Can you work these out from the model? Positions are in its coordinate system, mm. A direction names the side the tool comes from. Give positions to 0.01 mm unless a question says otherwise; leave off trailing zeros. Write each loop counter-clockwise with the first axis right and the second up, starting at its lowest first coordinate (ties: lowest second). Pieces come first, ordered by that corner, then holes.
1. Thinking about a two-plate mould opening in Z: for faces 3 (the cylindrical face through (-10.74, 1.48, -2.38)), 4 (the flat face through (3, 0, 0)), 5 (the cylindrical face through (-2.44, 6.59, -0.54)), which applies, pulls with the +Z half, pulls with the -Z half, needs draft (parallel to the pull), parting line crosses it, or undercut?
2. If I drill on probe 1 along X at (y, z) = (0.8, 0); probe 2 along Y at (x, z) = (-4, -3.5); probe 3 along X at (y, z) = (11, -1.5), over which ranges is the centre line in solid material (lowest first)?
3. On a 3-axis mill with a long thin cutter (end or side, diameter ignored), from which of +Z, -Z, +X, -X, +Y, -Y can I reach the whole of each face in a straight line? I mean faces 1 (the cylindrical face through (-4.88, 7.93, -1.08)), 2 (the flat face through (-2, 13, 2)). Say none if no direction works.
4. I'm going to push a flat-ended pin straight in: pin 1 (1 mm diameter, centred on y = 1.5, z = -5.5, fed in from -X). Where does the tip first touch, or does it pass through?
5. Suppose I cut it at D-D (y = 1). Please give me the cut outline in (x, z).
6. Suppose I cut it at A-A (z = 0). Please give me the cut outline in (x, y), and give its area (3 significant figures).
7. Suppose I cut it at C-C (z = -8). Please give me the cut outline in (x, y).
8. Suppose I cut it at B-B (x = -8). Please give me the cut outline in (y, z).
```python
from build123d import *

# Parameters (mm, degrees)
SKETCH_1_R          = 11
EXTRUDE_1_DEPTH     = 3
SKETCH_2_R          = 5
EXTRUDE_2_DEPTH     = 10
SKETCH_3_R          = 2.5
CUT_EXTRUDE_1_DEPTH = 13
SKETCH_4_R          = 1.5
CUT_EXTRUDE_2_DEPTH = 3


with BuildPart() as part:
    # 草图1 → 凸台-拉伸1 (new body)
    with BuildSketch(Plane(origin=(0, 0, 0), x_dir=(1, 0, 0), z_dir=(0, 1, 0))):
        with Locations(Location((0, 0, 0), (0, 0, 270))):
            Circle(SKETCH_1_R)
    extrude(amount=EXTRUDE_1_DEPTH)

    # 草图2 → 凸台-拉伸2 (add)
    with BuildSketch(Plane(origin=(0, 3, 0), x_dir=(1, 0, 0), z_dir=(0, 1, 0))):
        with Locations(Location((0, 0, 0), (0, 0, 270))):
            Circle(SKETCH_2_R)
    extrude(amount=EXTRUDE_2_DEPTH)

    # 草图3 → 切除-拉伸1 (cut)
    with BuildSketch(Plane(origin=(0, 13, 0), x_dir=(1, 0, 0), z_dir=(0, 1, 0))):
        with Locations(Location((0, 0, 0), (0, 0, 270))):
            Circle(SKETCH_3_R)
    extrude(amount=-CUT_EXTRUDE_1_DEPTH, mode=Mode.SUBTRACT)

    # 草图4 → 切除-拉伸2 (cut)
    with BuildSketch(Plane.XZ):
        with Locations(Location((0, 8, 0), (0, 0, 270))):
            Circle(SKETCH_4_R)
        with Locations(Location((8, 0, 0), (0, 0, 270))):
            Circle(SKETCH_4_R)
        with Locations(Location((0, -8, 0), (0, 0, 270))):
            Circle(SKETCH_4_R)
        with Locations(Location((-8, 0, 0), (0, 0, 270))):
            Circle(SKETCH_4_R)
    extrude(amount=-CUT_EXTRUDE_2_DEPTH, mode=Mode.SUBTRACT)


solid = part.part
```
Checks:
1. face 3: parting line crosses it
1. face 4: needs draft
1. face 5: undercut
2. probe 1: x = -11 to -9.5, -6.5 to -2.5, 2.5 to 6.5, 9.5 to 11
2. probe 2: y = 0 to 3
2. probe 3: x = -4.77 to -2, 2 to 4.77
3. face 1: +Y
3. face 2: +Z, -Z, +X, -X, +Y
4. pin 1: stops at x = -9.8
5. outline: circle Ø22 at (0, 0); hole circle Ø3 at (-8, 0); hole circle Ø5 at (0, 0); hole circle Ø3 at (0, -8); hole circle Ø3 at (0, 8); hole circle Ø3 at (8, 0)
6. outline: (-11, 0) - (-9.5, 0) - (-9.5, 3) - (-11, 3) - close; (-6.5, 0) - (-2.5, 0) - (-2.5, 13) - (-5, 13) - (-5, 3) - (-6.5, 3) - close; (2.5, 0) - (6.5, 0) - (6.5, 3) - (5, 3) - (5, 13) - (2.5, 13) - close; (9.5, 0) - (11, 0) - (11, 3) - (9.5, 3) - close
6. area: 83.0 mm2
7. outline: (-7.55, 0) - (-1.5, 0) - (-1.5, 3) - (-7.55, 3) - close; (1.5, 0) - (7.55, 0) - (7.55, 3) - (1.5, 3) - close
8. outline: (0, -7.55) - (3, -7.55) - (3, -1.5) - (0, -1.5) - close; (0, 1.5) - (3, 1.5) - (3, 7.55) - (0, 7.55) - close
